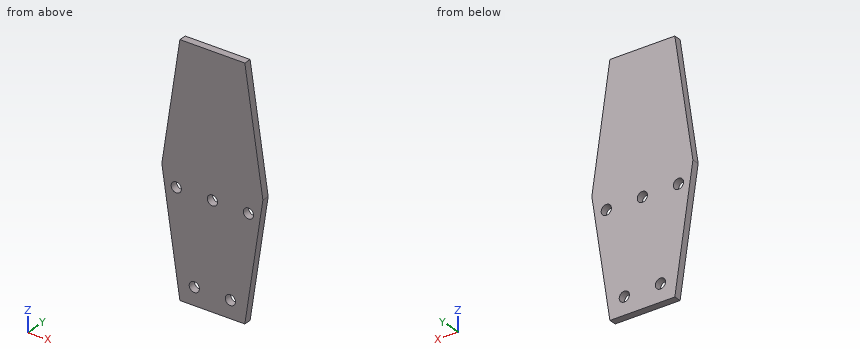
```python
from build123d import *

# Parameters (mm, degrees)
F0_R     = 3.5941
F1_DEPTH = 5.08


with BuildPart() as f1:
    # F0 (on Front) → F1 (new body)
    with BuildSketch(Plane.XZ):
        Polygon((-55.358764, -45.511816), (-45.198764, -45.511816), (-19.798764, -45.511816), (-9.638764, -45.511816), (3.061236, 39.743538), (-9.638764, 124.998892), (-19.798764, 124.998892), (-45.198764, 124.998892), (-55.358764, 124.998892), (-68.058764, 39.743538), align=None)
        with Locations((-45.198764, -33.317022)):
            Circle(F0_R, mode=Mode.SUBTRACT)
        with Locations((-57.898764, 27.551538)):
            Circle(F0_R, mode=Mode.SUBTRACT)
        with Locations((-19.798764, -33.317022)):
            Circle(F0_R, mode=Mode.SUBTRACT)
        with Locations((-32.498764, 27.551538)):
            Circle(F0_R, mode=Mode.SUBTRACT)
        with Locations((-7.098764, 27.551538)):
            Circle(F0_R, mode=Mode.SUBTRACT)
    extrude(amount=F1_DEPTH)


solid = f1.part
```
Source: CAD feature listing. Evaluate the final solid. Frame: model axes, mm. Give positions to 0.01 mm unless a question says otherwise; leave off trailing zeros. Loops run counter-clockwise (first coordinate to the right, second up) from the corner with the lowest first, then second, coordinate; pieces in that order, holes last. Notation, with made-up numbers: (32.5, -29.75) -> (46.5, -29.75) arc R18 cw to (46.5, -4.75) -> close; hole circle Ø10 at (-7.75, 78). An arc over 180 degrees is marked (long way). Use a Markdown table: item, result. Add a question column.
(1) Section query C-C (y = -4). Output: boundary loops of the cut face in (x, z), then the cut area to 3 significant figures.
(2) First-contact query: pin 1 Ø1.5 at (y, z) = (-3.5, 31.5) entering from +X. Flat tip, straight axial feed; report the tip coordinate or a pass-through.
(3) Ray query, line 1 (X direction, y = -2.3, z = -33); line 2 (Z direction, x = -19, y = -0.6); line 3 (X direction, y = -2.4, z = -36). Return the intervals inside material, ascending.
(4) Section query B-B (z = -35). Output: boundary loops of the cut face in (x, y).
(5) Section query D-D (x = -46). Output: boundary loops of the cut face in (y, z).
(6) Section query A-A (x = -33). Output: boundary loops of the cut face in (y, z).
Checked values:
| question | item | result |
|---|---|---|
| 1 | outline | (-68.06, 39.74) -> (-55.36, -45.51) -> (-9.64, -45.51) -> (3.06, 39.74) -> (-9.64, 125) -> (-55.36, 125) -> close; hole circle Ø7.19 at (-57.9, 27.55); hole circle Ø7.19 at (-45.2, -33.32); hole circle Ø7.19 at (-32.5, 27.55); hole circle Ø7.19 at (-19.8, -33.32); hole circle Ø7.19 at (-7.1, 27.55) |
| 1 | area | 9,760 mm^2 |
| 2 | pin 1 | x = 1.94 |
| 3 | line 1 | -57.22 to -48.78, -41.62 to -23.38, -16.22 to -7.77 |
| 3 | line 2 | -45.51 to -36.82, -29.81 to 125 |
| 3 | line 3 | -56.78 to -47.59, -42.81 to -22.19, -17.41 to -8.22 |
| 4 | outline | (-56.92, -5.08) -> (-48.37, -5.08) -> (-48.37, 0) -> (-56.92, 0) -> close; (-42.02, -5.08) -> (-22.97, -5.08) -> (-22.97, 0) -> (-42.02, 0) -> close; (-16.62, -5.08) -> (-8.07, -5.08) -> (-8.07, 0) -> (-16.62, 0) -> close |
| 5 | outline | (-5.08, -45.51) -> (0, -45.51) -> (0, -36.82) -> (-5.08, -36.82) -> close; (-5.08, -29.81) -> (0, -29.81) -> (0, 125) -> (-5.08, 125) -> close |
| 6 | outline | (-5.08, -45.51) -> (0, -45.51) -> (0, 23.99) -> (-5.08, 23.99) -> close; (-5.08, 31.11) -> (0, 31.11) -> (0, 125) -> (-5.08, 125) -> close |
